Print and shaded views of the part. All mm, measured from the part's lowest x, y and z. A direction names the side the tool comes from. Give positions to 0.01 mm unless a question says otherwise; leave off trailing zeros. Write each loop counter-clockwise with the first axis right and the second up, starting at its lowest first coordinate (ties: lowest second). Pieces come first, ordered by that corner, then holes.
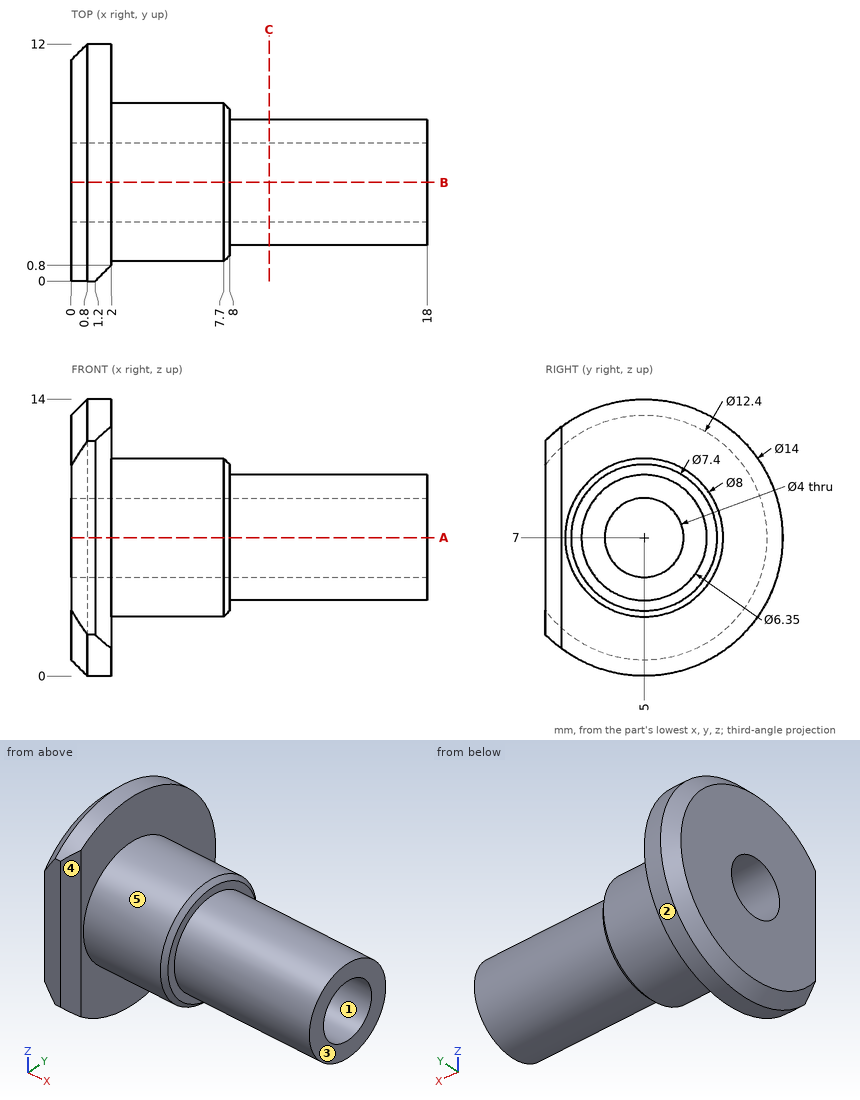
1. Drill centre lines: line 1 along Y through (x, z) = (5.25, 7); line 2 along Y through (x, z) = (9.25, 7) (3 decimals); line 3 along X through (y, z) = (10.5, 4.25). Where is each one in solid material? Low to high.
2. 3-axis set-ups, long thin cutter, end or side, ignore diameter. For the marked faces 4 and 5: which of +Z, -Z, +X, -X, +Y, -Y reach the whole face in a straight line?
3. Saw through at C-C on x = 10. Give the cut face in (y, z) (3 decimals).
4. Drop flat-ended pins along their axis: pin 1 (1 mm diameter, centred on x = 15, y = 3.5, fed in from -Z); pin 2 (5 mm diameter, centred on x = 4, z = 5, fed in from +Y). Give the stop position or say it passes through.
5. Saw through at B-B on y = 5. Give the cut face in (x, z) (3 decimals), plus the area to 3 significant figures.
6. Mould opens along Z. For the marked faces 1, 2 and 3 say: pulls with the +Z half, pulls with the -Z half, needs draft (parallel to the pull), parting line crosses it, or undercut.
7. Saw through at A-A on z = 7. Give the cut face in (x, y) (3 decimals).
Outcome:
1. line 1: y = 1 to 3, 7 to 9
1. line 2: y = 1.825 to 3, 7 to 8.175
1. line 3: x = 0 to 2
2. face 4: +Z, -Z, +X, -Y
2. face 5: +X
3. outline: circle Ø6.35 at (5, 7); hole circle Ø4 at (5, 7)
4. pin 1: stops at z = 3.99
4. pin 2: stops at y = 11.98
5. outline: (0, 0.8) - (0.8, 0) - (2, 0) - (2, 3) - (7.7, 3) - (8, 3.3) - (8, 3.825) - (18, 3.825) - (18, 5) - (0, 5) - close; (0, 9) - (18, 9) - (18, 10.175) - (8, 10.175) - (8, 10.7) - (7.7, 11) - (2, 11) - (2, 14) - (0.8, 14) - (0, 13.2) - close
5. area: 66.8 mm2
6. face 1: undercut
6. face 2: parting line crosses it
6. face 3: needs draft
7. outline: (0, 0) - (1.2, 0) - (2, 0.8) - (2, 1) - (7.7, 1) - (8, 1.3) - (8, 1.825) - (18, 1.825) - (18, 3) - (0, 3) - close; (0, 7) - (18, 7) - (18, 8.175) - (8, 8.175) - (8, 8.7) - (7.7, 9) - (2, 9) - (2, 12) - (0.8, 12) - (0, 11.2) - close
